Can you work these out from the model? Positions are in its coordinate system, mm. Face numbers are marked on the shaded views. Give positions to 0.01 mm unless a question says otherwise; leave off trailing zeros. Loops run counter-clockwise (first coordinate to the right, second up) from the corner with the lowest first, then second, coordinate; pieces in that order, holes last. Notation, with made-up numbers: M 49,8 L 54,8 A7 ccw 54,12 Z; hole C 16,-6.75 d3. An arc over 180 degrees is marked long. One line per item, written item: value. Start each with the question number.
from build123d import *

# Parameters (mm, degrees)
BOSS_EXTRUDE1_DEPTH      = 2
SKETCH1_3_W              = 70
SKETCH1_3_H              = 43
BOSS_EXTRUDE2_DEPTH      = 4
SKETCH1_5_W              = 40
SKETCH1_5_H              = 24
CUT_EXTRUDE4_DEPTH       = 2
CUT_EXTRUDE5_REACH       = 81.505
SKETCH2_W                = 39
SKETCH2_H                = 1.5
BOSS_EXTRUDE3_DEPTH      = 0.1
BOSS_EXTRUDE3_DEPTH_BACK = 0.5
FILLET1_R                = 1


with BuildPart() as part:
    # Sketch1 → Boss-Extrude1 (new body)
    with BuildSketch(Plane(origin=(0, 0, 0), x_dir=(1, 0, 0), z_dir=(0, 1, 0))):
        Polygon((0, 0), (64, 0), (64, -1), (66, -1), (66, -38), (64, -38), (64, -39), (0, -39), align=None)
    extrude(amount=BOSS_EXTRUDE1_DEPTH)

    # Sketch1<3> → Boss-Extrude2 (add)
    with BuildSketch(Plane(origin=(0, 0, 0), x_dir=(1, 0, 0), z_dir=(0, 1, 0))):
        with Locations((33, -19.5)):
            Rectangle(SKETCH1_3_W, SKETCH1_3_H)
        Polygon((0, 0), (64, 0), (64, -1), (66, -1), (66, -38), (64, -38), (64, -39), (0, -39), align=None, mode=Mode.SUBTRACT)
    extrude(amount=BOSS_EXTRUDE2_DEPTH)

    # Sketch1<5> → Cut-Extrude4 (cut)
    with BuildSketch(Plane(origin=(0, 0, 0), x_dir=(1, 0, 0), z_dir=(0, 1, 0))):
        with Locations((20, -27)):
            Rectangle(SKETCH1_5_W, SKETCH1_5_H)
        with BuildLine():
            ThreePointArc((40, -15), (52, -27), (40, -39))
            Line((40, -39), (40, -15))
        make_face()
    extrude(amount=CUT_EXTRUDE4_DEPTH, mode=Mode.SUBTRACT)

    # Sketch2 → Cut-Extrude5 (cut, up to next)
    with BuildSketch(Plane(origin=(0, 0, 0), x_dir=(0, 0, -1), z_dir=(1, 0, 0)), mode=Mode.PRIVATE) as cut_extrude5_sk1:
        with Locations((-19.5, 3.25)):
            Rectangle(SKETCH2_W, SKETCH2_H)
    cut_extrude5_tool1 = extrude(cut_extrude5_sk1.sketch, amount=-CUT_EXTRUDE5_REACH, mode=Mode.PRIVATE) & part.part
    add(cut_extrude5_tool1.solids().sort_by_distance((0, 3.25, 19.5))[0], mode=Mode.SUBTRACT)

    # Sketch3 → Boss-Extrude3 (add, two sides: drawn at the far end of the back side and taken through both)
    with BuildSketch(Plane(origin=(0, 4, 0), x_dir=(1, 0, 0), z_dir=(0, 1, 0)).offset(-BOSS_EXTRUDE3_DEPTH_BACK)):
        Polygon((-2, -41), (68, -41), (68, 2), (-2, 2), (-2, -1), (65, -1), (65, -38), (-2, -38), align=None)
    extrude(amount=BOSS_EXTRUDE3_DEPTH + BOSS_EXTRUDE3_DEPTH_BACK)

    # Fillet1
    fillet1_edges = [part.edges().sort_by_distance(p)[0] for p in [
        (33, 4.1, 41),
        (68, 4.1, 19.5),
        (33, 4.1, -2),
        (68, 2.05, -2),
        (-2, 0, 19.5),
        (-2, 2.05, -2),
        (33, 0, 41),
        (-2, 2.05, 41),
        (68, 2.05, 41),
        (33, 0, -2),
        (68, 0, 19.5),
    ]]
    fillet(fillet1_edges, radius=FILLET1_R)


solid = part.part
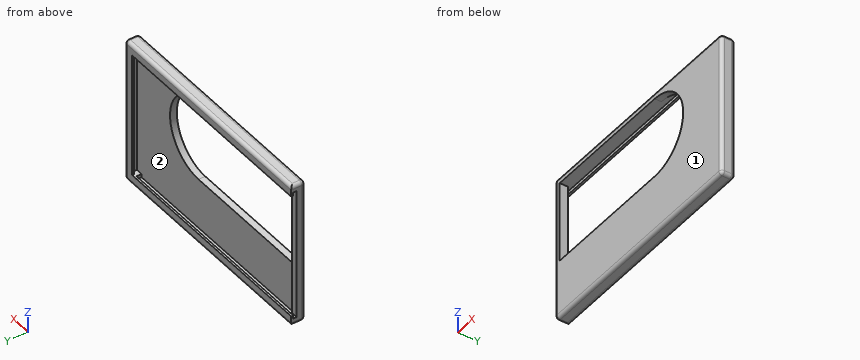
Q1. If we section it at B-B, the plane z = 27: Write out the boundary of the cut face in (x, y), plus the area to 3 significant figures.
Q2. For P1, Ø0.5, axis at y = 4, z = 25.5, coming from the -X side; P2, Ø0.8, axis at y = 3, z = 38.5, coming from the -X side; P3, Ø11.5, axis at x = 41, z = 13, coming from the +Y side, each with a flat end and sliding along its axis, tell me the tip position at first contact or that it passes through.
Q3. If we section it at D-D, the plane z = 12.5: Write out the boundary of the cut face in (x, y), plus the area to 3 significant figures.
Q4. If we section it at A-A, the plane x = 17: Write out the boundary of the cut face in (y, z), plus the area to 3 significant figures.
Q5. If we section it at C-C, the plane x = 56.5: Write out the boundary of the cut face in (y, z), plus the area to 3 significant figures.
Q6. If we mould it in two halves opening along X, with no side actions, what happens to the marked faces 1 and 2? For each: released by +X, released by -X, zero draft, split by the parting line, or undercut.
Q7. I need wall thicknesses on line 1 along Z through (x, y) = (6, 0.85); line 2 along Z through (x, y) = (63, 2.55); line 3 along X through (y, z) = (2.4, 16.5). Which ranges of each line are inside material? Lowest first, please.
Response:
1. outline: M -2,1 A1 ccw -1,0 L 0,0 L 0,2.5 L -2,2.5 Z; M 52,0 L 67,0 A1 ccw 68,1 L 68,3.1 A1 ccw 67,4.1 L 65,4.1 L 65,3.5 L 66,3.5 L 66,2 L 52,2 Z
1. area: 41.2 mm^2
2. P1: x = 65
2. P2: x = 64
2. P3: y = 2
3. outline: M -2,1 A1 ccw -1,0 L 67,0 A1 ccw 68,1 L 68,3.1 A1 ccw 67,4.1 L 65,4.1 L 65,3.5 L 66,3.5 L 66,2 L 0,2 L 0,2.5 L -2,2.5 Z
3. area: 145 mm^2
4. outline: M 0,-1 A1 ccw 1,-2 L 3.1,-2 A1 ccw 4.1,-1 L 4.1,1 L 3.5,1 L 3.5,0 L 2,0 L 2,15 L 0,15 Z; M 0,39 L 3.5,39 L 3.5,38 L 4.1,38 L 4.1,40 A1 ccw 3.1,41 L 1,41 A1 ccw 0,40 Z
4. area: 46.7 mm^2
5. outline: M 0,-1 A1 ccw 1,-2 L 3.1,-2 A1 ccw 4.1,-1 L 4.1,1 L 3.5,1 L 3.5,0 L 2,0 L 2,39 L 3.5,39 L 3.5,38 L 4.1,38 L 4.1,40 A1 ccw 3.1,41 L 1,41 A1 ccw 0,40 Z
5. area: 94.7 mm^2
6. face 1: zero draft
6. face 2: undercut
7. line 1: -1.99 to 15, 39 to 40.99
7. line 2: -2 to 0, 39 to 41
7. line 3: -2 to 0, 66 to 68
